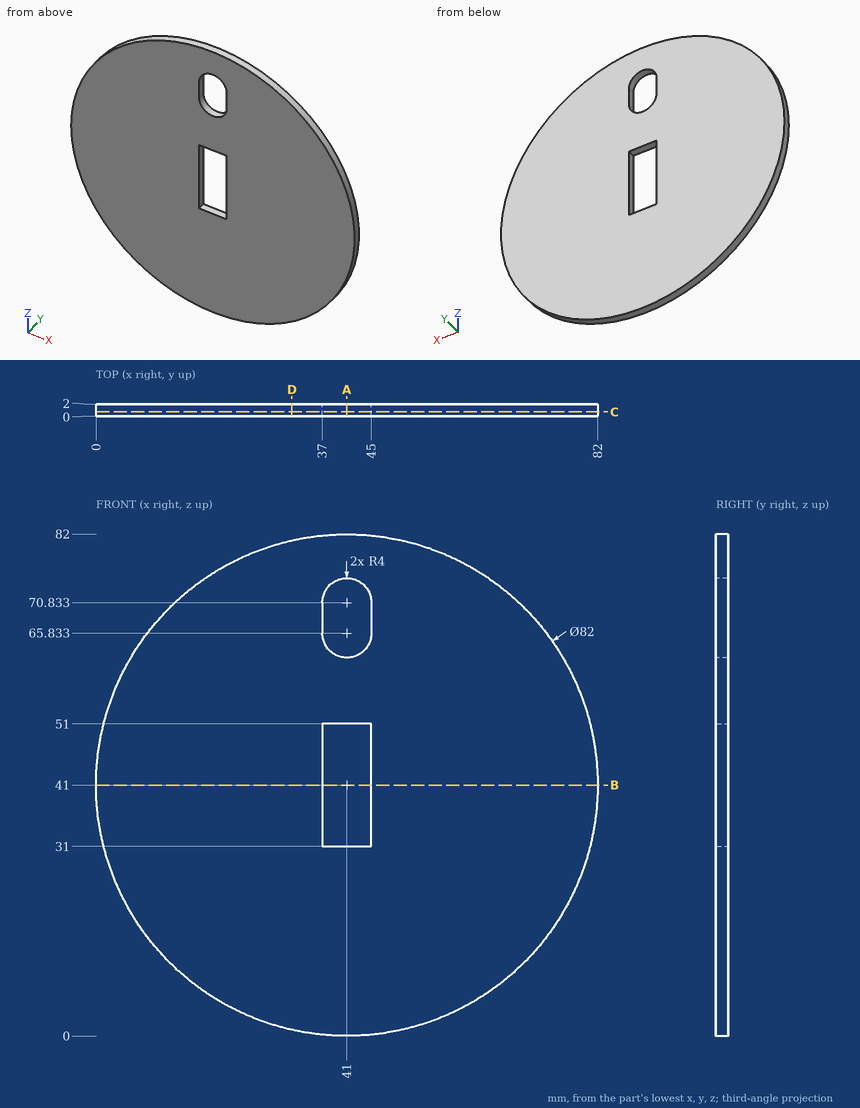
Design review of the part shown in the three views and the two pictorial views. Dimensions are in mm from the part's minimum x, y and z. Round coordinates to 2 decimals unless told otherwise and drop trailing zeros. Write each loop counter-clockwise with the first axis right and the second up, starting at its lowest first coordinate (ties: lowest second). Pieces come first, ordered by that corner, then holes. Notation, with made-up numbers: (89, 60) - (128, 60) arc R22 ccw to (128, 67) - close; hole circle Ø7 at (63.5, 27). An arc over 180 degrees is marked (long way). Write item = value, one per line. Start each with the question number.
1. Consider section A-A on x = 41. State the section outline as (y, z) points.
2. Consider section D-D on x = 32. State the section outline as (y, z) points.
3. Wall thickness on L1, parallel to X at y = 0.5, z = 74 (1 decimal); L2, parallel to X at y = 1.3, z = 50.5 (1 decimal); L3, parallel to Z at x = 16, y = 1.45 (1 decimal): over which ranges is each line inside the solid? List them lowest first.
4. For pin 1 Ø1 at (x, y) = (39, 1.5) entering from -Z; pin 2 Ø1 at (y, z) = (1, 68) entering from -X (1 decimal); pin 3 Ø0.6 at (x, y) = (42.5, 1) entering from +Z, all flat-tipped, find the tip position at first contact; note any pin that passes through.
5. Consider section B-B on z = 41. State the section outline as (x, y) points, plus the area to 3 significant figures.
6. Consider section C-C on y = 0.7. State the section outline as (x, z) points, plus the area to 3 significant figures.
Evaluation:
q1.outline = (0, 0) - (2, 0) - (2, 31) - (0, 31) - close; (0, 51) - (2, 51) - (2, 61.83) - (0, 61.83) - close; (0, 74.83) - (2, 74.83) - (2, 82) - (0, 82) - close
q2.outline = (0, 1) - (2, 1) - (2, 81) - (0, 81) - close
q3.L1 = 16.7 to 38.6, 43.4 to 65.3
q3.L2 = 1.1 to 37, 45 to 80.9
q3.L3 = 8.5 to 73.5
q4.pin_1 = 0.03
q4.pin_2 = 9.7
q4.pin_3 = 81.98
q5.outline = (0, 0) - (37, 0) - (37, 2) - (0, 2) - close; (45, 0) - (82, 0) - (82, 2) - (45, 2) - close
q5.area = 148 mm2
q6.outline = circle Ø82 at (41, 41); hole (37, 31) - (45, 31) - (45, 51) - (37, 51) - close; hole (37, 65.83) arc R4 ccw to (45, 65.83) - (45, 70.83) arc R4 ccw to (37, 70.83) - close
q6.area = 5,030 mm2
